Could you check a few things on this model? Use its own coordinates, in mm. A direction names the side the tool comes from. Coordinates: 2 decimals unless noted, no trailing zeros. Write each loop counter-clockwise with the first axis right and the second up, starting at its lowest first coordinate (ties: lowest second). Pieces come first, ordered by that corner, then holes.
Autodesk Inventor part; units mm, degrees
ref_plane "YZ Plane" through (0, 0, 0) normal (1, 0, 0) x (0, 1, 0)
ref_plane "XZ Plane" through (0, 0, 0) normal (0, 1, 0) x (-1, 0, 0)
ref_plane "XY Plane" through (0, 0, 0) normal (0, 0, 1) x (1, 0, 0)
sketch "Sketch1" plane through (0, 0, 0) normal (1, 0, 0) x (0, 1, 0)
  line L0 (0, 0) -> (69.85, 0)
  line L1 (69.85, 0) -> (69.85, -150.4)
  line L2 (69.85, -150.4) -> (0, -150.4)
  line L3 (0, -150.4) -> (0, 0)
  dimension "d0" = 69.85
  dimension "d1" = 150.4
extrude "Extrusion1" add sketch "Sketch1" along normal blind 2
sketch "Sketch2" plane through (2, 0, 0) normal (1, 0, 0) x (0, 0, -1)
  line L0 (150.4, 0) -> (150.4, 69.85)
  line L1 (150.4, 69.85) -> (0, 69.85)
  line L2 (0, 69.85) -> (0, 0)
  line L3 (0, 0) -> (150.4, 0)
  line L4 (150.4, 69.85) -> (148.4, 69.85)
  line L5 (148.4, 69.85) -> (148.4, 0)
  line L6 (148.4, 0) -> (150.4, 0)
  line L7 (150.4, 0) -> (150.4, 69.85)
  line L8 (0, 69.85) -> (2, 69.85)
  line L9 (2, 69.85) -> (2, 0)
  line L10 (2, 0) -> (0, 0)
  line L11 (0, 0) -> (0, 69.85)
  line L12 (0, 0) -> (150.4, 0)
  line L13 (150.4, 0) -> (150.4, 2)
  line L14 (150.4, 2) -> (0, 2)
  line L15 (0, 2) -> (0, 0)
  point P0 (2, 2)
  point P1 (148.4, 2)
  dimension "d4" = 2
  dimension "d5" = 2
  dimension "d6" = 2
extrude "Extrusion2" add sketch "Sketch2" along normal blind 2 contours L14 L9 L1 L5
sketch "Sketch3" plane through (4, 0, 0) normal (1, 0, 0) x (0, 0, -1)
  line L0 (150.4, 0) -> (150.4, 69.85)
  line L1 (0, 0) -> (150.4, 0)
  line L2 (0, 69.85) -> (0, 0)
  line L3 (150.4, 69.85) -> (0, 69.85)
  line L4 (0, 69.85) -> (75.2, 69.85) construction
  line L5 (75.2, 69.85) -> (75.2, 0) construction
  line L6 (75.2, 0) -> (0, 0) construction
  line L7 (0, 0) -> (0, 69.85) construction
  line L8 (0, 0) -> (150.4, 0) construction
  line L9 (0, 0) -> (37.6, 0) construction
  line L10 (37.6, 0) -> (37.6, 69.85) construction
  line L11 (37.6, 69.85) -> (0, 69.85) construction
  line L12 (0, 69.85) -> (0, 0) construction
  line L13 (150.4, 0) -> (150.4, 69.85) construction
  line L14 (75.2, 69.85) -> (150.4, 69.85) construction
  line L15 (150.4, 69.85) -> (150.4, 0) construction
  line L16 (150.4, 0) -> (75.2, 0) construction
  line L17 (75.2, 0) -> (75.2, 69.85) construction
  line L18 (75.2, 0) -> (112.8, 0) construction
  line L19 (112.8, 0) -> (112.8, 69.85) construction
  line L20 (112.8, 69.85) -> (75.2, 69.85) construction
  line L21 (75.2, 69.85) -> (75.2, 0) construction
  line L22 (34.425, 0) -> (34.425, 69.85) construction
  line L23 (34.425, 69.85) -> (40.775, 69.85) construction
  line L24 (40.775, 69.85) -> (40.775, 0) construction
  line L25 (40.775, 0) -> (34.425, 0) construction
  line L26 (34.425, 0) -> (40.775, 69.85) construction
  line L27 (34.425, 69.85) -> (40.775, 0) construction
  line L28 (72.025, 0) -> (72.025, 69.85) construction
  line L29 (72.025, 69.85) -> (78.375, 69.85) construction
  line L30 (78.375, 69.85) -> (78.375, 0) construction
  line L31 (78.375, 0) -> (72.025, 0) construction
  line L32 (72.025, 0) -> (78.375, 69.85) construction
  line L33 (72.025, 69.85) -> (78.375, 0) construction
  line L34 (109.625, 0) -> (109.625, 69.85) construction
  line L35 (109.625, 69.85) -> (115.975, 69.85) construction
  line L36 (115.975, 69.85) -> (115.975, 0) construction
  line L37 (115.975, 0) -> (109.625, 0) construction
  line L38 (109.625, 0) -> (115.975, 69.85) construction
  line L39 (109.625, 69.85) -> (115.975, 0) construction
  line L40 (34.425, 69.85) -> (40.775, 69.85)
  line L41 (40.775, 69.85) -> (40.775, 0)
  line L42 (40.775, 0) -> (34.425, 0)
  line L43 (34.425, 0) -> (34.425, 69.85)
  line L44 (72.025, 0) -> (78.375, 0)
  line L45 (78.375, 0) -> (78.375, 69.85)
  line L46 (78.375, 69.85) -> (72.025, 69.85)
  line L47 (72.025, 69.85) -> (72.025, 0)
  line L48 (109.625, 69.85) -> (115.975, 69.85)
  line L49 (115.975, 69.85) -> (115.975, 0)
  line L50 (115.975, 0) -> (109.625, 0)
  line L51 (109.625, 0) -> (109.625, 69.85)
  point P0 (37.6, 34.925)
  point P1 (75.2, 34.925)
  point P2 (112.8, 34.925)
  dimension "d9" = 6.35
  dimension "d10" = 6.35
  dimension "d11" = 6.35
extrude "Extrusion3" add sketch "Sketch3" along normal blind 4 contours L1 L51 L3 L49 | L1 L47 L3 L45 | L1 L43 L3 L41
sketch "Sketch4" plane through (0, 69.85, 0) normal (0, 1, 0) x (1, 0, 0)
  line L0 (0, 150.4) -> (0, 0)
  line L1 (0, 150.4) -> (0, 0) construction
  line L2 (0, 0) -> (2, 0) construction
  line L3 (2, 2) -> (2, 0) construction
  line L4 (2, 2) -> (4, 2) construction
  line L5 (4, 34.425) -> (4, 2) construction
  line L6 (4, 34.425) -> (8, 34.425) construction
  line L7 (8, 40.775) -> (8, 34.425) construction
  line L8 (4, 40.775) -> (8, 40.775) construction
  line L9 (4, 72.025) -> (4, 40.775) construction
  line L10 (4, 72.025) -> (8, 72.025) construction
  line L11 (8, 78.375) -> (8, 72.025) construction
  line L12 (4, 78.375) -> (8, 78.375) construction
  line L13 (4, 109.625) -> (4, 78.375) construction
  line L14 (4, 109.625) -> (8, 109.625) construction
  line L15 (8, 115.975) -> (8, 109.625) construction
  line L16 (4, 115.975) -> (8, 115.975) construction
  line L17 (4, 148.4) -> (4, 115.975) construction
  line L18 (2, 148.4) -> (4, 148.4) construction
  line L19 (2, 150.4) -> (2, 148.4) construction
  line L20 (0, 150.4) -> (2, 150.4) construction
  line L21 (2, 0) -> (0, 0)
  line L22 (0, 0) -> (0, 150.4)
  line L23 (0, 150.4) -> (2, 150.4)
  line L24 (2, 150.4) -> (2, 0)
  line L25 (2, 0) -> (8, 0)
  line L26 (8, 0) -> (8, 150.4)
  line L27 (8, 150.4) -> (2, 150.4)
  line L28 (2, 150.4) -> (2, 0)
extrude "Extrusion4" cut sketch "Sketch4" against normal blind 2 contours L27 L26 L25 L24
sketch "Sketch5" plane through (0, 67.85, 0) normal (0, 1, 0) x (1, 0, 0)
  line L0 (4, 115.975) -> (8, 115.975)
  line L1 (4, 148.4) -> (4, 115.975)
  line L2 (2, 148.4) -> (4, 148.4)
  line L3 (2, 2) -> (2, 148.4)
  line L4 (4, 2) -> (2, 2)
  line L5 (4, 34.425) -> (4, 2)
  line L6 (8, 34.425) -> (4, 34.425)
  line L7 (8, 40.775) -> (8, 34.425)
  line L8 (4, 40.775) -> (8, 40.775)
  line L9 (4, 72.025) -> (4, 40.775)
  line L10 (8, 72.025) -> (4, 72.025)
  line L11 (8, 78.375) -> (8, 72.025)
  line L12 (4, 78.375) -> (8, 78.375)
  line L13 (4, 109.625) -> (4, 78.375)
  line L14 (8, 109.625) -> (4, 109.625)
  line L15 (8, 115.975) -> (8, 109.625)
  line L16 (2, 2) -> (4, 2)
  line L17 (2, 2) -> (8, 2)
  line L18 (8, 2) -> (8, 148.4)
  line L19 (8, 148.4) -> (2, 148.4)
  line L20 (2, 148.4) -> (2, 2)
  point P0 (0, 0)
  point P1 (4, 2)
extrude "Extrusion5" add sketch "Sketch5" against normal blind 2 contours L1 L19 L18 L0 | L18 L12 L13 L14 | L18 L8 L9 L10 | L5 L6 L18 L17
sketch "Sketch7" plane through (4, 0, 0) normal (-1, 0, 0) x (0, 0, 1)
  line L0 (-109.625, 2) -> (-115.975, 2)
  line L1 (-115.975, 0) -> (-115.975, 2)
  line L2 (-109.625, 0) -> (-115.975, 0)
  line L3 (-109.625, 2) -> (-109.625, 0)
  line L4 (-72.025, 2) -> (-78.375, 2)
  line L5 (-78.375, 0) -> (-78.375, 2)
  line L6 (-72.025, 0) -> (-78.375, 0)
  line L7 (-72.025, 2) -> (-72.025, 0)
  line L8 (-34.425, 2) -> (-40.775, 2)
  line L9 (-40.775, 0) -> (-40.775, 2)
  line L10 (-34.425, 0) -> (-40.775, 0)
  line L11 (-34.425, 2) -> (-34.425, 0)
  point P0 (0, 0)
extrude "Extrusion6" add sketch "Sketch7" along normal blind 2
sketch "Sketch8" plane through (0, 67.85, 0) normal (0, 1, 0) x (1, 0, 0)
  line L0 (8, 2) -> (8, 148.4) construction
  line L1 (2, 148.4) -> (8, 148.4) construction
  line L2 (2, 2) -> (2, 148.4) construction
  line L3 (8, 2) -> (2, 2) construction
  line L4 (8, 34.425) -> (2, 34.425) construction
  line L5 (2, 34.425) -> (2, 40.775) construction
  line L6 (2, 40.775) -> (8, 40.775) construction
  line L7 (8, 40.775) -> (8, 34.425) construction
  circle A0 centre (5, 37.6) radius 2.25 construction
  line L8 (2, 2) -> (2, 148.4) construction
  line L9 (8, 109.625) -> (2, 109.625) construction
  line L10 (2, 109.625) -> (2, 115.975) construction
  line L11 (2, 115.975) -> (8, 115.975) construction
  line L12 (8, 115.975) -> (8, 109.625) construction
  circle A1 centre (5, 112.8) radius 2.25 construction
  circle A2 centre (5, 37.6) radius 2.25
  circle A3 centre (5, 112.8) radius 2.25
  point P0 (0, 0)
  point P1 (8, 72.025)
  point P2 (8, 78.375)
  dimension "d20" = 4.5
  dimension "d21" = 4.5
extrude "Extrusion7" cut sketch "Sketch8" against normal blind 5
properties part number "leftwall"
1. If we mould it in two halves opening along X, with no side actions, what happens to faces 1 (the face through (4.71, 65.38, -115.03)), 2 (the face through (5, 62.85, -113)), 3 (the face through (5, 67.85, -76)), 4 (the face through (4, 34, -94))? For each: pulls with the +X half, pulls with the -X half, needs draft (parallel to the pull), parting line crosses it, or undercut.
Verdict:
face 1: undercut
face 2: undercut
face 3: needs draft
face 4: pulls with the +X half
2. I want a section at A-A on y = 29. Please give me the cut outline in (x, z) (3 decimals).
Verdict:
outline: (0, -150.4) - (2, -150.4) - (2, -148.4) - (4, -148.4) - (4, -115.975) - (8, -115.975) - (8, -109.625) - (4, -109.625) - (4, -78.375) - (8, -78.375) - (8, -72.025) - (4, -72.025) - (4, -40.775) - (8, -40.775) - (8, -34.425) - (4, -34.425) - (4, -2) - (2, -2) - (2, 0) - (0, 0) - close
3. I want a section at B-B on z = -112.8. Please give me the cut outline in (x, y), plus the area to 3 significant figures.
Verdict:
outline: (0, 0) - (8, 0) - (8, 67.85) - (7.25, 67.85) - (7.25, 62.85) - (2.75, 62.85) - (2.75, 67.85) - (2, 67.85) - (2, 69.85) - (0, 69.85) - close
area: 524 mm2
4. For pin 1 (5 mm diameter, centred on y = 12.5, z = -92, fed in from +X); pin 2 (1.6 mm diameter, centred on x = 3.5, z = -23.5, fed in from -Y); pin 3 (1.8 mm diameter, centred on x = 4, y = 24.5, fed in from +Z), each with a flat end and sliding along its axis, tell me the tip position at first contact or that it passes through.
Verdict:
pin 1: stops at x = 4
pin 2: stops at y = 2
pin 3: stops at z = -2
5. Please list where these lines run through material, in increasing order: line 1 along Z through (x, y) = (5, 65.5) (3 decimals); line 2 along Z through (x, y) = (6.25, 5.5) (3 decimals); line 3 along X through (y, z) = (64.05, -37.6).
Verdict:
line 1: z = -115.975 to -115.05, -110.55 to -109.625, -78.375 to -72.025, -40.775 to -39.85, -35.35 to -34.425
line 2: z = -115.975 to -109.625, -78.375 to -72.025, -40.775 to -34.425
line 3: x = 0 to 2.75, 7.25 to 8
6. On a 3-axis mill with a long thin cutter (end or side, diameter ignored), from which of +Z, -Z, +X, -X, +Y, -Y can I reach the whole of each face in a straight line? I mean faces 5 (the face through (3, 38, -148.4)), 6 (the face through (4, 34, -56)), 7 (the face through (4, 34, -132)), 8 (the face through (0, 34, -74)), 9 (the face through (6, 65.85, -18)). Say none if no direction works.
Verdict:
face 5: -Z, +X, +Y, -Y
face 6: +X, -Y
face 7: -Z, +X, -Y
face 8: +Z, -Z, -X, +Y, -Y
face 9: +Z, +X, -Y
7. I want a section at C-C on z = -133.5. Please give me the cut outline in (x, y).
Verdict:
outline: (0, 0) - (2, 0) - (2, 2) - (4, 2) - (4, 65.85) - (8, 65.85) - (8, 67.85) - (2, 67.85) - (2, 69.85) - (0, 69.85) - close
8. I want a section at D-D on z = -73.5. Please give me the cut outline in (x, y).
Verdict:
outline: (0, 0) - (8, 0) - (8, 67.85) - (2, 67.85) - (2, 69.85) - (0, 69.85) - close
